For this review, take the finished solid that the model builds, in its own axes (mm). A direction names the side the tool comes from. Coordinates: 2 decimals unless noted, no trailing zeros. Write each loop counter-clockwise with the first axis right and the second up, starting at its lowest first coordinate (ties: lowest second). Pieces come first, ordered by that corner, then holes. Notation, with made-up numbers: M 52,11.25 L 75,11.25 A7 cw 75,20.25 Z; hole C 27.25,28 d1. An arc over 180 degrees is marked long. Return JSON: item names as keys, results as strings.
```python
from build123d import *

# Parameters (mm, degrees)
SKETCH1_W           = 90
SKETCH1_H           = 50
BOSS_EXTRUDE1_DEPTH = 21
CUT_EXTRUDE1_DEPTH  = 16
SKETCH4_R           = 2.5
CUT_EXTRUDE2_DEPTH  = 63.626624678
SKETCH5_W           = 10
SKETCH5_H           = 6.2
CUT_EXTRUDE3_DEPTH  = 19
SKETCH6_R           = 3
CUT_EXTRUDE4_DEPTH  = 20
SKETCH11_R          = 1.5
BOSS_EXTRUDE3_DEPTH = 3
BOSS_EXTRUDE2_DEPTH = 23.630686795
CUT_EXTRUDE6_DEPTH  = 19
SKETCH17_W          = 16
SKETCH17_H          = 3.2
CUT_EXTRUDE10_DEPTH = 37.549476
SKETCH15_R          = 1.8
CUT_EXTRUDE8_DEPTH  = 1.5
SKETCH16_R          = 1.25
CUT_EXTRUDE9_DEPTH  = 19
CUT_EXTRUDE11_REACH = 23
SKETCH19_R          = 4
CHAMFER1_SIZE       = 8
CHAMFER2_SIZE       = 2
CUT_EXTRUDE12_REACH = 52
SKETCH21_W          = 21.5
SKETCH21_H          = 3
BOSS_EXTRUDE4_DEPTH = 5.5
CUT_EXTRUDE13_REACH = 23
SKETCH23_W          = 37.630686795
SKETCH23_H          = 16
SKETCH25_R          = 1.15
CUT_EXTRUDE14_DEPTH = 10
SKETCH26_R          = 1
CUT_EXTRUDE15_DEPTH = 36.75
SKETCH27_W          = 2.5
SKETCH27_H          = 25
BOSS_EXTRUDE6_DEPTH = 6.5
SKETCH28_W          = 10
SKETCH28_H          = 0.8
CUT_EXTRUDE16_DEPTH = 4
SKETCH22_R          = 2
SKETCH22_R_2        = 0.8
BOSS_EXTRUDE7_DEPTH = 3


with BuildPart() as part:
    # Sketch1 → Boss-Extrude1 (new body)
    with BuildSketch(Plane(origin=(0, 0, 0), x_dir=(1, 0, 0), z_dir=(0, 1, 0))):
        with Locations((-5, 0)):
            Rectangle(SKETCH1_W, SKETCH1_H)
    extrude(amount=BOSS_EXTRUDE1_DEPTH)

    # Sketch2 → Cut-Extrude1 (cut)
    with BuildSketch(Plane(origin=(0, 21, 0), x_dir=(1, 0, 0), z_dir=(0, 1, 0))):
        Polygon((-44.5, 10.75), (3.5, 10.75), (13.5, 5), (13.5, -5), (3.5, -10.75), (-44.5, -10.75), align=None)
    extrude(amount=-CUT_EXTRUDE1_DEPTH, mode=Mode.SUBTRACT)

    # Sketch4 → Cut-Extrude2 (cut, through all)
    with BuildSketch(Plane(origin=(0, 3.891653574, -38.585684316), x_dir=(1, 0, 0), z_dir=(0, 0.545410535, 0.838169045))):
        Circle(SKETCH4_R)
    cut_extrude2 = extrude(amount=CUT_EXTRUDE2_DEPTH, mode=Mode.SUBTRACT)

    # Sketch5 → Cut-Extrude3 (cut)
    with BuildSketch(Plane(origin=(0, 29, 0), x_dir=(1, 0, 0), z_dir=(0, 0.545410535, 0.838169045))):
        with Locations((0, 0.013708289)):
            Rectangle(SKETCH5_W, SKETCH5_H)
    cut_extrude3 = extrude(amount=-CUT_EXTRUDE3_DEPTH, mode=Mode.SUBTRACT)

    # Sketch6 → Cut-Extrude4 (cut)
    with BuildSketch(Plane(origin=(0, 3.891653574, -38.585684316), x_dir=(1, 0, 0), z_dir=(0, 0.545410535, 0.838169045))):
        Circle(SKETCH6_R)
    cut_extrude4 = extrude(amount=CUT_EXTRUDE4_DEPTH, mode=Mode.SUBTRACT)

    # Sketch11 → Boss-Extrude3 (add)
    with BuildSketch(Plane(origin=(0, 5, 0), x_dir=(1, 0, 0), z_dir=(0, 1, 0))):
        with Locations((-36.5, 0)):
            Circle(SKETCH11_R)
        Polygon((11.3, 6.265), (11.3, -6.265), (13.5, -5), (13.5, 5), align=None)
    extrude(amount=BOSS_EXTRUDE3_DEPTH)

    # Sketch9 → Boss-Extrude2 (add)
    with BuildSketch(Plane.ZY.offset(-13.5)):
        Polygon((-8, 18.7), (-8, 15.5), (-6, 15.5), (-6, 14.7), (-10.75, 13.6), (-11.152370245, 13.6), (-11.152370245, 14.662668332), (-11.152370245, 18.060784345), (-6.635479906, 21), (0, 21), (0, 18.7), align=None)
    boss_extrude2 = extrude(amount=BOSS_EXTRUDE2_DEPTH)

    # Mirror1: Cut-Extrude2, Cut-Extrude3, Cut-Extrude4, Boss-Extrude2 across plane
    add(cut_extrude2.mirror(Plane.XY), mode=Mode.SUBTRACT)
    add(cut_extrude3.mirror(Plane.XY), mode=Mode.SUBTRACT)
    add(cut_extrude4.mirror(Plane.XY), mode=Mode.SUBTRACT)
    add(boss_extrude2.mirror(Plane.XY))

    # Sketch10 → Cut-Extrude6 (cut)
    with BuildSketch(Plane(origin=(0, 21, 0), x_dir=(1, 0, 0), z_dir=(0, 1, 0))):
        Polygon((-44.5, 12.5), (-44.5, 23), (-8, 23), (-8, 12.55), (-10.049475977, 12.55), (-10.049475977, 10.75), (-44.5, 10.75), (-44.5, 0), (-50, 0), (-50, 12.5), align=None)
        Polygon((8, 25), (8, 10.75), (28.5, 10.75), (28.5, 4), (46.328078386, 4), (46.328078386, 30.717572765), (8, 31.044325351), align=None)
    cut_extrude6 = extrude(amount=-CUT_EXTRUDE6_DEPTH, mode=Mode.SUBTRACT)

    # Mirror2: Cut-Extrude6 across plane
    add(cut_extrude6.mirror(Plane.XY), mode=Mode.SUBTRACT)

    # Sketch17 → Cut-Extrude10 (cut)
    with BuildSketch(Plane.ZY.offset(10.049475977)):
        with Locations((0, 17.1)):
            Rectangle(SKETCH17_W, SKETCH17_H)
    extrude(amount=-CUT_EXTRUDE10_DEPTH, mode=Mode.SUBTRACT)

    # Sketch15 → Cut-Extrude8 (cut)
    with BuildSketch(Plane(origin=(0, 21, 0), x_dir=(1, 0, 0), z_dir=(0, 1, 0))):
        with Locations((35, 0)):
            Circle(SKETCH15_R)
    extrude(amount=-CUT_EXTRUDE8_DEPTH, mode=Mode.SUBTRACT)

    # Sketch16 → Cut-Extrude9 (cut)
    with BuildSketch(Plane(origin=(0, 21, 0), x_dir=(1, 0, 0), z_dir=(0, 1, 0))):
        with Locations((-47.5, 19)):
            Circle(SKETCH16_R)
        with Locations((-47.5, -19)):
            Circle(SKETCH16_R)
    extrude(amount=-CUT_EXTRUDE9_DEPTH, mode=Mode.SUBTRACT)

    # Sketch19 → Cut-Extrude11 (cut, up to next)
    with BuildSketch(Plane(origin=(0, 21, 0), x_dir=(1, 0, 0), z_dir=(0, 1, 0)), mode=Mode.PRIVATE) as cut_extrude11_sk1:
        Circle(SKETCH19_R)
    cut_extrude11_tool1 = extrude(cut_extrude11_sk1.sketch, amount=-CUT_EXTRUDE11_REACH, mode=Mode.PRIVATE) & part.part
    add(cut_extrude11_tool1.solids().sort_by_distance((0, 21, 0))[0], mode=Mode.SUBTRACT)

    # Chamfer1
    chamfer1_edges = [part.edges().sort_by_distance(p)[0] for p in [
        (-44.5, 2, -17.75),
        (-44.5, 2, 17.75),
    ]]
    chamfer(chamfer1_edges, length=CHAMFER1_SIZE)

    # Chamfer2
    chamfer2_edges = [part.edges().sort_by_distance(p)[0] for p in [
        (40, 1, -25),
        (40, 1, 25),
    ]]
    chamfer(chamfer2_edges, length=CHAMFER2_SIZE)

    # Sketch20 → Cut-Extrude12 (cut, up to next)
    with BuildSketch(Plane.XY.offset(25), mode=Mode.PRIVATE) as cut_extrude12_sk1:
        Polygon((-28.5, 15.5), (-22, 15.5), (-22, 15.9), (-16.5, 15.9), (-16.5, 15.5), (-10, 15.5), (-10, 21), (-28.5, 21), (-28.5, 15.8), align=None)
    cut_extrude12_tool1 = extrude(cut_extrude12_sk1.sketch, amount=-CUT_EXTRUDE12_REACH, mode=Mode.PRIVATE) & part.part
    add(cut_extrude12_tool1.solids().sort_by_distance((-19.25, 18.306354, 25))[0], mode=Mode.SUBTRACT)

    # Sketch21 → Boss-Extrude4 (add)
    with BuildSketch(Plane.ZY.offset(44.5)):
        with Locations((0, 3.5)):
            Rectangle(SKETCH21_W, SKETCH21_H)
    extrude(amount=BOSS_EXTRUDE4_DEPTH)

    # Sketch23 → Cut-Extrude13 (cut, up to next)
    with BuildSketch(Plane(origin=(0, 21, 0), x_dir=(1, 0, 0), z_dir=(0, 1, 0)), mode=Mode.PRIVATE) as cut_extrude13_sk1:
        with Locations((8.684656602, 0)):
            Rectangle(SKETCH23_W, SKETCH23_H)
    cut_extrude13_tool1 = extrude(cut_extrude13_sk1.sketch, amount=-CUT_EXTRUDE13_REACH, mode=Mode.PRIVATE) & part.part
    add(cut_extrude13_tool1.solids().sort_by_distance((8.684657, 21, 0))[0], mode=Mode.SUBTRACT)

    # Sketch25 → Cut-Extrude14 (cut)
    with BuildSketch(Plane(origin=(0, 21, 0), x_dir=(1, 0, 0), z_dir=(0, 1, 0))):
        with Locations((29, 0)):
            Circle(SKETCH25_R)
    extrude(amount=-CUT_EXTRUDE14_DEPTH, mode=Mode.SUBTRACT)

    # Sketch26 → Cut-Extrude15 (cut, through all)
    with BuildSketch(Plane.XY.offset(10.75)):
        with Locations((11.80251356, 10.471486046)):
            Circle(SKETCH26_R)
    extrude(amount=-CUT_EXTRUDE15_DEPTH, mode=Mode.SUBTRACT)

    # Sketch27 → Boss-Extrude6 (add)
    with BuildSketch(Plane(origin=(0, 2, 0), x_dir=(1, 0, 0), z_dir=(0, 1, 0))):
        with Locations((-48.75, 0)):
            Rectangle(SKETCH27_W, SKETCH27_H)
    extrude(amount=BOSS_EXTRUDE6_DEPTH)

    # Sketch28 → Cut-Extrude16 (cut)
    with BuildSketch(Plane(origin=(0, 17.786458912, 11.573944585), x_dir=(1, 0, 0), z_dir=(0, 0.838169045, 0.545410535))):
        with Locations((0, -2.783094473)):
            Rectangle(SKETCH28_W, SKETCH28_H)
    cut_extrude16 = extrude(amount=-CUT_EXTRUDE16_DEPTH, mode=Mode.SUBTRACT)

    # Mirror3: Cut-Extrude16 across plane
    add(cut_extrude16.mirror(Plane.XY), mode=Mode.SUBTRACT)

    # Sketch22 → Boss-Extrude7 (add)
    with BuildSketch(Plane(origin=(0, 5, 0), x_dir=(1, 0, 0), z_dir=(0, 1, 0))):
        with Locations((-42.3, -5.65)):
            Circle(SKETCH22_R)
        with Locations((-42.3, -5.65)):
            Circle(SKETCH22_R_2, mode=Mode.SUBTRACT)
        with Locations((9.66, 4.95)):
            Circle(SKETCH22_R)
        with Locations((9.66, 4.95)):
            Circle(SKETCH22_R_2, mode=Mode.SUBTRACT)
    extrude(amount=BOSS_EXTRUDE7_DEPTH)


solid = part.part
```
1. Draft analysis for pull direction Y (two halves, no side actions). For faces 5 (the face through (-0.07, 15.984, 14.199)), 6 (the face through (18, 12, 10.75)), 7 (the face through (35, 19.5, 0)), state which applies: +Y half, -Y half, draft (parallel to the pull), parting line (faces both ways), or undercut.
Checks:
{"face 5": "undercut", "face 6": "draft", "face 7": "+Y half"}
2. We need section C-C (z = 0). State the section outline as (x, y) points.
Checks:
{"outline": "M -50,0 L 40,0 L 40,21 L 36.8,21 L 36.8,19.5 L 33.2,19.5 L 33.2,21 L 30.15,21 L 30.15,11 L 27.85,11 L 27.85,21 L 27.5,21 L 27.5,15.5 L 13.5,15.5 L 13.5,8 L 11.3,8 L 11.3,5 L -35,5 L -35,8 L -38,8 L -38,5 L -47.5,5 L -47.5,8.5 L -50,8.5 Z"}
3. We need section D-D (x = -13). State the section outline as (y, z) points, plus the area to 4 significant figures.
Checks:
{"outline": "M 0,-25 L 21,-25 L 21,-23 L 2,-23 L 2,-10.75 L 5,-10.75 L 5,10.75 L 2,10.75 L 2,23 L 15.5,23 L 15.5,25 L 0,25 Z", "area": "229.5 mm2"}
4. We need section A-A (y = 4). Give the number of separate pieces and of enclosed holes in the cut face, plus the area to 3 significant figures.
Checks:
{"separate pieces": "1", "enclosed holes": "4", "area": "2,650 mm2"}
5. Clearance check with flat-ended pins moving along their axes: pin 1 Ø4 at (x, z) = (-26, -5.5) entering from -Y; pin 2 Ø0.6 at (x, z) = (-11.5, 24.5) entering from +Y; pin 3 Ø7 at (y, z) = (7, -18) entering from +X; pin 4 Ø3 at (x, z) = (-42, 6) entering from +Y. State where each tip first meets the part, or that it passes through.
Checks:
{"pin 1": "y = 0", "pin 2": "y = 15.5", "pin 3": "x = 8", "pin 4": "y = 8"}
6. For faces 1 (the face through (-9, 12, 12.55)), 2 (the face through (-45, 21, 20)), 3 (the face through (27.5, 18, 0)), 4 (the face through (24, 2, -17)), list the 3-axis set-ups (+Z, -Z, +X, -X, +Y, -Y) from which the entire face can be reached by the end or side of a thin tool; tool diameter is ignored.
Checks:
{"face 1": "+Y", "face 2": "+Z, -Z, +X, -X, +Y", "face 3": "-X, +Y", "face 4": "-Z, +X, +Y"}
7. Wall thickness on L1, parallel to X at y = 15, z = -21.5; L2, parallel to X at y = 7.35, z = 5.65; L3, parallel to X at y = 20.4, z = 0: over which ranges is each line inside the solid? List them lowest first. Write a range as from..to.
Checks:
{"L1": "-50..-44.5, -8..-2.5, 2.5..8", "L2": "-50..-47.5, -44.3..-43.1, -41.5..-40.3, 11.3..28.5", "L3": "27.5..27.85, 30.15..33.2, 36.8..40"}
8. We need section B-B (x = -4). State the section outline as (y, z) points.
Checks:
{"outline": "M 0,-25 L 21,-25 L 21,-17.46 L 12.7,-12.06 L 13.13,-11.39 L 16.49,-13.57 L 20.11,-8 L 15.5,-8 L 15.5,-6 L 14.7,-6 L 13.6,-10.75 L 5,-10.75 L 5,10.75 L 13.6,10.75 L 14.7,6 L 15.5,6 L 15.5,8 L 20.11,8 L 16.49,13.57 L 13.13,11.39 L 12.7,12.06 L 21,17.46 L 21,25 L 0,25 Z"}
